The listing builds one solid part. Answer for the finished solid, in the listing's coordinates (mm). A direction names the side the tool comes from. Round coordinates to 2 decimals unless told otherwise and drop trailing zeros. Order: outer loops, then holes, each group sorted by start corner. A loop starts at its lowest first (then second) coordinate and runs counter-clockwise, first axis right, second up. Notation, with made-up numbers: (-21, -34.75) - (2, -34.75) arc R24 cw to (2, 4.25) - close; hole circle Ø1 at (-17.75, -22.75). An arc over 180 degrees is marked (long way). Use CSV: the item, a comma, the result in double quotes. Start each with the question number.
Item 1: Find section B-B, the plane x = 219.25. Give the vertices of the cut face in (y, z), plus the area to 3 significant figures.
Item 2: Straight lines are drawn through the part: line 1 along Y through (x, z) = (236.25, 10); line 2 along X through (y, z) = (110, 1.5); line 3 along Y through (x, z) = (230.75, 1.75). For each, find the intervals that lie inside material, in ascending order. Write a range as [from, to].
Item 3: Find section D-D, the plane x = 225.25. Give the vertices of the cut face in (y, z), plus the area to 3 significant figures.
Item 4: Flat-ended cylindrical pins translate along their axes: P1, Ø12.5, axis at x = 228, y = 107.5, coming from the -Z side; P2, Ø7, axis at x = 233.32, y = 73.2, coming from the +Z side; P3, Ø3, axis at x = 226.5, z = 9.5, coming from the -Y side; P4, Ø5, axis at x = 220.5, y = 110.5, coming from the -Z side. Find the tip coordinate at first contact, or state that the pin passes through.
Item 5: For faces 1 (the flat face through (226, 85.901, 9)), 2 (the cylindrical face through (212.225, 64.625, 3.131)), 3 (the cylindrical face through (232.664, 106.156, 5.635)), determine the directions among +Z, -Z, +X, -X, +Y, -Y from which every point of the face is accessible in a straight line to the end or side of a thin tool.
Item 6: Find section C-C, the plane y = 72. Give the vertices of the cut face in (x, z).
Item 7: Find section A-A, the plane z = 5. Count the separate pieces of the cut face and the enclosed holes in it, plus the area to 3 significant figures.
```python
from build123d import *

# Parameters (mm, degrees)
SKETCH1_R           = 2.9845
SKETCH1_R_2         = 7.9502
SKETCH1_R_3         = 1.524
SKETCH1_R_4         = 7.250000001
BOSS_EXTRUDE1_DEPTH = 12.7
SKETCH1_3_R         = 7.9502
SKETCH1_3_R_2       = 7.250000001
CUT_EXTRUDE1_DEPTH  = 11.43
CUT_EXTRUDE2_START  = 6.35
SKETCH1_4_R         = 2.9845
CUT_EXTRUDE2_DEPTH  = 6.35


with BuildPart() as part:
    # Sketch1 → Boss-Extrude1 (new body)
    # profile 1 of 3: a face of its own
    with BuildSketch(Plane.XY):
        with BuildLine():
            ThreePointArc((211.319871652, 66.845549451), (212.249807622, 64.60048542), (214.494871652, 63.670549451))
            Line((214.494871652, 63.670549451), (236.144871651, 63.670549451))
            ThreePointArc((236.144871651, 63.670549451), (238.389935682, 64.60048542), (239.319871651, 66.845549451))
            Line((239.319871651, 66.845549451), (239.319871651, 85.900629451))
            Line((239.319871651, 85.900629451), (211.319871652, 85.900629451))
            Line((211.319871652, 85.900629451), (211.319871652, 66.845549451))
        make_face()
        with Locations((217.319871651, 73.200629451)):
            Circle(SKETCH1_R, mode=Mode.SUBTRACT)
        with Locations((233.319871652, 73.200629451)):
            Circle(SKETCH1_R, mode=Mode.SUBTRACT)
    # profile 2 of 3: a face of its own
    with BuildSketch(Plane.XY):
        with BuildLine():
            Line((211.319871652, 111.26550139), (211.319871652, 85.900629451))
            Line((211.319871652, 85.900629451), (239.319871651, 85.900629451))
            Line((239.319871651, 85.900629451), (239.319871651, 117.025629451))
            ThreePointArc((239.319871651, 117.025629451), (238.389935682, 119.270693481), (236.144871651, 120.200629451))
            Line((236.144871651, 120.200629451), (220.254999713, 120.200629451))
            ThreePointArc((220.254999713, 120.200629451), (219.039979814, 119.958946966), (218.009935681, 119.27069348))
            Line((218.009935681, 119.27069348), (212.24980762, 113.510565419))
            ThreePointArc((212.24980762, 113.510565419), (211.561554136, 112.480521287), (211.319871652, 111.26550139))
        make_face()
        with Locations((225.31987165, 109.200629449)):
            Circle(SKETCH1_R_2, mode=Mode.SUBTRACT)
        with Locations((236.11487165, 109.200629449)):
            Circle(SKETCH1_R_3, mode=Mode.SUBTRACT)
    # profile 3 of 3: a face of its own
    with BuildSketch(Plane.XY):
        with Locations((225.31987165, 109.200629449)):
            Circle(SKETCH1_R_2)
        with Locations((225.31987165, 109.200629449)):
            Circle(SKETCH1_R_4, mode=Mode.SUBTRACT)
    extrude(amount=BOSS_EXTRUDE1_DEPTH)

    # Sketch1<3> → Cut-Extrude1 (cut)
    with BuildSketch(Plane.XY):
        with Locations((225.31987165, 109.200629449)):
            Circle(SKETCH1_3_R)
        with Locations((225.31987165, 109.200629449)):
            Circle(SKETCH1_3_R_2, mode=Mode.SUBTRACT)
    extrude(amount=CUT_EXTRUDE1_DEPTH, mode=Mode.SUBTRACT)

    # Sketch1<4> → Cut-Extrude2 (cut)
    with BuildSketch(Plane.XY.offset(CUT_EXTRUDE2_START)):
        with BuildLine():
            ThreePointArc((211.319871652, 66.845549451), (212.249807622, 64.60048542), (214.494871652, 63.670549451))
            Line((214.494871652, 63.670549451), (236.144871651, 63.670549451))
            ThreePointArc((236.144871651, 63.670549451), (238.389935682, 64.60048542), (239.319871651, 66.845549451))
            Line((239.319871651, 66.845549451), (239.319871651, 85.900629451))
            Line((239.319871651, 85.900629451), (211.319871652, 85.900629451))
            Line((211.319871652, 85.900629451), (211.319871652, 66.845549451))
        make_face()
        with Locations((217.319871651, 73.200629451)):
            Circle(SKETCH1_4_R, mode=Mode.SUBTRACT)
        with Locations((233.319871652, 73.200629451)):
            Circle(SKETCH1_4_R, mode=Mode.SUBTRACT)
    extrude(amount=CUT_EXTRUDE2_DEPTH, mode=Mode.SUBTRACT)


solid = part.part
```
Worked out:
1,outline,"(63.67, 0) - (70.92, 0) - (70.92, 6.35) - (63.67, 6.35) - close; (75.48, 0) - (104.07, 0) - (104.07, 11.43) - (105.24, 11.43) - (105.24, 12.7) - (85.9, 12.7) - (85.9, 6.35) - (75.48, 6.35) - close; (113.17, 11.43) - (114.34, 11.43) - (114.34, 0) - (120.04, 0) - (120.04, 12.7) - (113.17, 12.7) - close"
1,area,"418 mm²"
2,line 1,"y = [85.9, 107.68], [110.72, 120.2]"
2,line 2,"x = [211.32, 217.41], [233.23, 234.82], [237.41, 239.32]"
2,line 3,"y = [63.67, 71.68], [74.72, 103.39], [115.01, 120.2]"
3,outline,"(63.67, 0) - (101.25, 0) - (101.25, 11.43) - (101.95, 11.43) - (101.95, 12.7) - (85.9, 12.7) - (85.9, 6.35) - (63.67, 6.35) - close; (116.45, 11.43) - (117.15, 11.43) - (117.15, 0) - (120.2, 0) - (120.2, 12.7) - (116.45, 12.7) - close"
3,area,"377 mm²"
4,P1,"stops at z = 0"
4,P2,"stops at z = 6.35"
4,P3,"stops at y = 85.9"
4,P4,"stops at z = 11.43"
5,face 1,"+Z, +X, -X, -Y"
5,face 2,"+Z, -Z, -X, -Y"
5,face 3,"-Z"
6,outline,"(211.32, 0) - (214.59, 0) - (214.59, 6.35) - (211.32, 6.35) - close; (220.05, 0) - (230.59, 0) - (230.59, 6.35) - (220.05, 6.35) - close; (236.05, 0) - (239.32, 0) - (239.32, 6.35) - (236.05, 6.35) - close"
7,separate pieces,"1"
7,enclosed holes,"4"
7,area,"1,290 mm²"
